Design review of the part built by this model. Coordinates are the model's own, in mm. A direction names the side the tool comes from. Coordinates: 2 decimals unless noted, no trailing zeros. Loops run counter-clockwise (first coordinate to the right, second up) from the corner with the lowest first, then second, coordinate; pieces in that order, holes last. Notation, with made-up numbers: (77.5, 1) - (92.5, 1) arc R22 ccw to (92.5, 37) - close; hole circle Ø1 at (46.5, -29.5). An arc over 180 degrees is marked (long way). Answer in a Markdown table with one row per item. Add a question column.
(1) Clearance check with flat-ended pins moving along their axes: pin 1 (1 mm diameter, centred on x = 0, z = 8, fed in from +Y); pin 2 (6 mm diameter, centred on x = 5.5, z = 10, fed in from -Y); pin 3 (5 mm diameter, centred on x = -12, z = 2, fed in from -Y). State where each tip first meets the part, or that it passes through.
(2) The part is to be moulded in two halves that separate along X. For faces 1 (the face through (-2.012, 15.324, -0.74)), 2 (the face through (5.76, -9.25, 8.11)), 3 (the face through (8.715, -6.54, 8.112)), 4 (the face through (-6, -3, 16)), say which applies: released by +X, released by -X, zero draft, split by the parting line, or undercut.
(3) We need section A-A, the plane y = 1.5. Write out the cut boundary in (x, z).
(4) For faces 5 (the face through (0, -7, -1.5)), 6 (the face through (5.6, -3.3, 7.4)), 7 (the face through (10.49, -2.95, 8.11)), list the 3-axis set-ups (+Z, -Z, +X, -X, +Y, -Y) from which the entire face can be reached by the end or side of a thin tool; tool diameter is ignored.
(5) To check wall thickness, follow L1, parallel to Y at x = -11, z = 6.75; L2, parallel to X at y = -11, z = 8.75; L3, parallel to X at y = -12, z = 14. State the ranges of each line that lie inside material, in increasing order. Write a range as [from, to].
from build123d import *

# Parameters (mm, degrees)
F2_R            = 12.9556701783
F3_DEPTH        = 16
F5_DEPTH        = 16
F5_COPIES_COUNT = 17
F8_R            = 15.4556701783
F8_R_2          = 12.9556701783
F9_DEPTH        = 1.5
F10_DEPTH       = 17.501


# Not quite as in the source:
# - a feature of the source that left no trace in its solid (it failed there, or was rolled back) is left out
# - a pattern or mirror of a feature is missing from the dataset's text; its kind, count and spacing are read off the source's solid


with BuildPart() as f3:
    # F2 (on Top) → F3 (new body)
    with BuildSketch(Plane.XY):
        Circle(F2_R)
    extrude(amount=F3_DEPTH)

    # F4 (on face) → F5 (cut, through all)
    with BuildSketch(Plane.XY.offset(16)):
        with BuildLine():
            ThreePointArc((-2.019679411, 12.797276462), (-1.6609629062, 12.6980751446), (-1.4996370898, 12.362676258))
            ThreePointArc((-1.4996370898, 12.362676258), (0, 10.8956701783), (1.4996370898, 12.362676258))
            ThreePointArc((1.4996370898, 12.362676258), (1.6609629062, 12.6980751446), (2.019679411, 12.797276462))
            ThreePointArc((2.019679411, 12.797276462), (0, 12.9556701783), (-2.019679411, 12.797276462))
        make_face()
    f5 = extrude(amount=-F5_DEPTH, mode=Mode.SUBTRACT)

    # F5_copies: F5 ×17 about axis
    f5_copies_axis = Axis((0, 0, 0), (0, 0, 1))
    for i in range(1, F5_COPIES_COUNT):
        add(f5.rotate(f5_copies_axis, i * 360 / F5_COPIES_COUNT), mode=Mode.SUBTRACT)

    # F8 (on face) + F2 (on Top) → F9 (join)
    with BuildSketch(Plane.XY):
        Circle(F8_R)
        Circle(F8_R_2, mode=Mode.SUBTRACT)
    with BuildSketch(Plane.XY):
        Circle(F2_R)
    extrude(amount=-F9_DEPTH)

    # F7 (on face) → F10 (cut, through all)
    with BuildSketch(Plane.XY.offset(16)):
        Polygon((3.7527767497, 6.5), (-3.7527767497, 6.5), (-7.5055534995, 0), (-3.7527767497, -6.5), (3.7527767497, -6.5), (7.5055534995, 0), align=None)
    extrude(amount=-F10_DEPTH, mode=Mode.SUBTRACT)


solid = f3.part
Responses:
| question | item | result |
|---|---|---|
| 1 | pin 1 | stops at y = 10.98 |
| 1 | pin 2 | stops at y = -12.23 |
| 1 | pin 3 | stops at y = -11.34 |
| 2 | face 1 | split by the parting line |
| 2 | face 2 | undercut |
| 2 | face 3 | undercut |
| 2 | face 4 | zero draft |
| 3 | outline | (-15.38, -1.5) - (-6.64, -1.5) - (-6.64, 16) - (-10.89, 16) - (-10.89, 0) - (-15.38, 0) - close; (6.64, -1.5) - (15.38, -1.5) - (15.38, 0) - (10.89, 0) - (10.89, 16) - (6.64, 16) - close |
| 4 | face 5 | -Z, +X, -X, +Y, -Y |
| 4 | face 6 | +Z, -Z |
| 4 | face 7 | +Z |
| 5 | L1 | y = [-6.34, -4.58], [-2.21, 0.48], [1.81, 4.03] |
| 5 | L2 | x = [-5.1, -3.2], [-1.36, 1.36], [3.2, 5.1] |
| 5 | L3 | x = [-4.88, -3.79], [-0.79, 0.79], [3.79, 4.88] |
